```python
from build123d import *

# Parameters (mm, degrees)
F0_R     = 1.5
F1_DEPTH = 2
F0_W     = 4
F0_H     = 7
F2_DEPTH = 0.1
F3_DEPTH = 1.9
F4_W     = 20
F4_H     = 3
F5_DEPTH = 0.1
F4_W_2   = 15.2
F6_DEPTH = 0.1


with BuildPart() as f1:
    # F0 (on Top) → F1 (new body)
    with BuildSketch(Plane.XY):
        Polygon((-20, 26.5), (-33, 26.5), (-33, 19.5), (-29, 19.5), (-29, 12.5), (-33, 12.5), (-33, -26.5), (-20, -26.5), (33, -26.5), (33, -23.5), (36.198911, -22.0798), (36.284242, 10.5), (34.509105, 13.5), (34.509105, 24.5), (33, 26.5), align=None)
        with Locations((-18.304507, -24)):
            Circle(F0_R, mode=Mode.SUBTRACT)
        with Locations((33.657469, -20.717213)):
            Circle(F0_R, mode=Mode.SUBTRACT)
        with Locations((-18.304507, 24)):
            Circle(F0_R, mode=Mode.SUBTRACT)
        with Locations((33.600888, 10.583145)):
            Circle(F0_R, mode=Mode.SUBTRACT)
    extrude(amount=F1_DEPTH)

    # F0 (on Top) → F2 (cut)
    with BuildSketch(Plane.XY):
        with Locations((-31, 16)):
            Rectangle(F0_W, F0_H)
    extrude(amount=-F2_DEPTH, mode=Mode.SUBTRACT)

    # F0 (on Top) → F3 (join)
    with BuildSketch(Plane.XY):
        with Locations((-31, 16)):
            Rectangle(F0_W, F0_H)
    extrude(amount=F3_DEPTH)

    # F4 (on face) → F5 (cut)
    with BuildSketch(Plane.XY.offset(2)):
        with Locations((2.509105, 24)):
            Rectangle(F4_W, F4_H)
        with Locations((23.509105, 24)):
            Rectangle(F4_W, F4_H)
    extrude(amount=-F5_DEPTH, mode=Mode.SUBTRACT)

    # F4 (on face) → F6 (cut)
    with BuildSketch(Plane.XY.offset(2)):
        with Locations((8.2, -24)):
            Rectangle(F4_W_2, F4_H)
        with Locations((24.4, -24)):
            Rectangle(F4_W_2, F4_H)
    extrude(amount=-F6_DEPTH, mode=Mode.SUBTRACT)


solid = f1.part
```
For this review, take the finished solid that the model builds, in its own axes (mm). A direction names the side the tool comes from. Round coordinates to 2 decimals unless told otherwise and drop trailing zeros. Write each loop counter-clockwise with the first axis right and the second up, starting at its lowest first coordinate (ties: lowest second). Pieces come first, ordered by that corner, then holes. Notation, with made-up numbers: M 6.5,0.25 L 42.5,0.25 A9 cw 42.5,13.25 Z; hole C 28,69.5 d5. An arc over 180 degrees is marked long. One line per item, written item: value. Start each with the question number.
(1) We need section A-A (z = 1.1). Give the boundary of the cut face in (x, y), and give its area (3 significant figures).
(2) Wall thickness on line 1 (X direction, y = 10.5, z = 0.2); line 2 (X direction, y = 12.5, z = 0.95); line 3 (X direction, y = -20.5, z = 0.7): over which ranges is each line inside the solid? List them lowest first.
(3) Machinability: for faces 1 (the flat face through (24, -24, 1.9)), 2 (the flat face through (33, -25, 1)), 3 (the flat face through (-33, 0, 1)), 4 (the flat face through (-31, 16, 1.9)), which of the approach directions +Z, -Z, +X, -X, +Y, -Y give a long, thin tool a straight path to every point of the face, cutting with its end or side? Answer none if there is none.
(4) Insertion check: pin 1 (1 mm diameter, centred on y = -18.5, z = 0.5, fed in from +X); pin 2 (0.9 mm diameter, centred on x = 24, y = -24, fed in from +Z). Each pin has a flat end and moves straight along its axis. Give the tip position at first contact, or say it passes through.
Result:
1. outline: M -33,-26.5 L 33,-26.5 L 33,-23.5 L 36.2,-22.08 L 36.28,10.5 L 34.51,13.5 L 34.51,24.5 L 33,26.5 L -33,26.5 Z; hole C -18.3,-24 d3; hole C -18.3,24 d3; hole C 33.6,10.58 d3; hole C 33.66,-20.72 d3
1. area: 3,600 mm²
2. line 1: -33 to 32.1, 35.1 to 36.28
2. line 2: -33 to 35.1
2. line 3: -33 to 32.17, 35.14 to 36.2
3. face 1: +Z
3. face 2: +Z, -Z, +X, -Y
3. face 3: +Z, -Z, -X, +Y, -Y
3. face 4: +Z, -X
4. pin 1: x = 36.21
4. pin 2: z = 1.9
